from build123d import *

# Parameters (mm, degrees)
SKETCH1_R           = 4
BOSS_EXTRUDE1_DEPTH = 3


with BuildPart() as part:
    # Sketch1 → Boss-Extrude1 (new body)
    with BuildSketch(Plane(origin=(0, 0, 0), x_dir=(1, 0, 0), z_dir=(0, 1, 0))):
        Polygon((4.965212315, 0), (2.482606158, 4.3), (-2.482606158, 4.3), (-4.965212315, 0), (-2.482606158, -4.3), (2.482606158, -4.3), align=None)
        Circle(SKETCH1_R, mode=Mode.SUBTRACT)
    extrude(amount=BOSS_EXTRUDE1_DEPTH)

    # Sketch2 → Revolve-Thin1 (revolve)
    with BuildSketch(Plane.XY):
        with BuildLine():
            ThreePointArc((0, 7.1), (2.899137803, 5.899137803), (4.1, 3))
            Line((4.1, 3), (0, 3))
            Line((0, 3), (0, 4))
            Line((0, 4), (2.93428015, 4))
            ThreePointArc((2.93428015, 4), (1.804161855, 5.520912533), (0, 6.1))
            Line((0, 6.1), (0, 7.1))
        make_face()
    revolve(axis=Axis((0, 7.455, 0), (0, -1, 0)))


solid = part.part
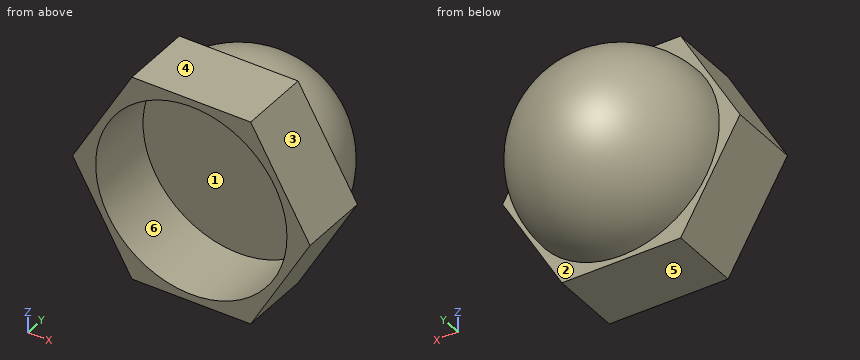
The listing builds one solid part. Answer for the finished solid, in the listing's coordinates (mm). Face numbers are marked on the shaded views. A direction names the side the tool comes from. Give positions to 0.01 mm unless a question says otherwise; leave off trailing zeros. Write each loop counter-clockwise with the first axis right and the second up, starting at its lowest first coordinate (ties: lowest second). Pieces come first, ordered by that corner, then holes.
Item 1: Section B-B, the plane z = 2.75 is taken. Write down the section's boundary in (x, y), plus the area to 3 significant figures.
Item 2: Section D-D, the plane y = 5.25 is taken. Write down the section's boundary in (x, z).
Item 3: Section C-C, the plane z = -3.5 is taken. Write down the section's boundary in (x, y), plus the area to 3 significant figures.
Item 4: Section A-A, the plane x = 0 is taken. Write down the section's boundary in (y, z), plus the area to 3 significant figures.
Item 5: Which of the six approach directions +Z, -Z, +X, -X, +Y, -Y give full straight-line access (tool end or side, diameter ignored) to the marked faces 1, 2 and 3?
Item 6: Find the intervals of material crossed by line 1 along Z through (x, y) = (0, 1.05); line 2 along Y through (x, z) = (2, -2); line 3 along Z through (x, y) = (-1, 1.5), in increasing order.
Item 7: Determine the mould class of the marked faces 4, 5 and 6 for opening direction Z: released by +Z, released by -Z, zero draft, split by the parting line, or undercut.
Item 8: Flat-ended cylindrical pins translate along their axes: P1, Ø2, axis at y = 1, z = 1.5, coming from the +X side; P2, Ø2, axis at x = 2.5, z = 0, coming from the -Y side; P3, Ø2.5, axis at x = -1, z = 2, coming from the +Y side. Find the tip coordinate at first contact, or state that the pin passes through.
Completed:
1. outline: (-3.38, 0) - (-2.9, 0) - (-2.9, 3) - (2.9, 3) - (2.9, 0) - (3.38, 0) - (3.38, 3) - (3.04, 3) arc R3.04 ccw to (-3.04, 3) - (-3.38, 3) - close; hole (-1.02, 4) - (1.02, 4) arc R1.43 ccw to start
1. area: 16.8 mm2
2. outline: circle Ø6.85 at (0, 0); hole circle Ø4.26 at (0, 0)
3. outline: (-2.94, 0) - (-1.94, 0) - (-1.94, 3) - (1.94, 3) - (1.94, 0) - (2.94, 0) - (2.94, 3) - (2.14, 3) arc R2.14 ccw to (-2.14, 3) - (-2.94, 3) - close
3. area: 13.2 mm2
4. outline: (0, -4.3) - (3, -4.3) - (3, -4.1) arc R4.1 ccw to (3, 4.1) - (3, 4.3) - (0, 4.3) - (0, 4) - (3, 4) - (3, -4) - (0, -4) - close; hole (4, -2.93) arc R3.1 ccw to (4, 2.93) - close
4. area: 19.2 mm2
5. face 1: -Y
5. face 2: +Y
5. face 3: +Z, +X, +Y, -Y
6. line 1: z = -4.3 to -4, 4 to 4.3
6. line 2: y = 3 to 4, 4.27 to 5.97
6. line 3: z = -4.3 to -3.87, 3.87 to 4.3
7. face 4: released by +Z
7. face 5: released by -Z
7. face 6: undercut
8. P1: stops at x = 4.68
8. P2: stops at y = 3
8. P3: stops at y = 6.98
